from build123d import *

# Parameters (mm, degrees)
SKETCH1_W                = 20
SKETCH1_H                = 30
BOSS_EXTRUDE1_DEPTH      = 10
BOSS_EXTRUDE2_DEPTH      = 20
BOSS_EXTRUDE2_DEPTH_BACK = 20
SKETCH2_R                = 2
BOSS_EXTRUDE3_DEPTH      = 5.08
BOSS_EXTRUDE3_DEPTH_BACK = 5.08
SKETCH4_R                = 2.413
SKETCH5_W                = 5.08
SKETCH5_H                = 10
CUT_EXTRUDE1_DEPTH       = 35.777069342


with BuildPart() as part:
    # Sketch1 → Boss-Extrude1 (new body)
    with BuildSketch(Plane(origin=(0, 0, 0), x_dir=(1, 0, 0), z_dir=(0, 1, 0))):
        Rectangle(SKETCH1_W, SKETCH1_H)
    extrude(amount=BOSS_EXTRUDE1_DEPTH)

    # Sketch2 → Boss-Extrude2 (add, two sides: drawn at the far end of the back side and taken through both)
    with BuildSketch(Plane.XY.offset(-BOSS_EXTRUDE2_DEPTH_BACK)):
        with Locations((0, 5)):
            Circle(SKETCH2_R)
    extrude(amount=BOSS_EXTRUDE2_DEPTH + BOSS_EXTRUDE2_DEPTH_BACK)

    # Sketch4 → Boss-Extrude3 (add, two sides: drawn at the far end of the back side and taken through both)
    with BuildSketch(Plane(origin=(0, 0, 0), x_dir=(0, 0, -1), z_dir=(1, 0, 0)).offset(-BOSS_EXTRUDE3_DEPTH_BACK)):
        with BuildLine():
            Line((-27, 9.826), (-20, 9.826))
            Line((-20, 9.826), (-20, 0.174))
            Line((-20, 0.174), (-27, 0.174))
            ThreePointArc((-27, 0.174), (-31.826, 5), (-27, 9.826))
        make_face()
        with Locations((-27, 5)):
            Circle(SKETCH4_R, mode=Mode.SUBTRACT)
    extrude(amount=BOSS_EXTRUDE3_DEPTH + BOSS_EXTRUDE3_DEPTH_BACK)

    # Sketch5 → Cut-Extrude1 (cut, through all)
    with BuildSketch(Plane(origin=(0, 9.826, 0), x_dir=(1, 0, 0), z_dir=(0, 1, 0))):
        with Locations((0, -26.826)):
            Rectangle(SKETCH5_W, SKETCH5_H)
    extrude(amount=-CUT_EXTRUDE1_DEPTH, mode=Mode.SUBTRACT)


solid = part.part
Verification items for the finished model (mm, model axes). A direction names the side the tool comes from. Give positions to 0.01 mm unless a question says otherwise; leave off trailing zeros. Loops run counter-clockwise (first coordinate to the right, second up) from the corner with the lowest first, then second, coordinate; pieces in that order, holes last.
1) Depth check by flat-ended pin: pin 1 Ø1.5 at (x, z) = (4.5, -14.5) entering from -Y; pin 2 Ø2 at (x, z) = (-1.5, 22) entering from -Y; pin 3 Ø4 at (y, z) = (7, 19.5) entering from +X; pin 4 Ø3 at (y, z) = (3, 27) entering from -X. Enter the tip coordinate at first touch or a pass-through.
2) Thickness scan on line 1 along Z through (x, y) = (3.35, 5); line 2 along Y through (x, z) = (-4.1, 27); line 3 along X through (y, z) = (1, 22.5). Record the ranges inside material, lowest first.
3) Sectioned sample at A-A, the plane y = 3.5. Enter the section's corners in (x, z).
4) Set-up check for faces 1 (the flat face through (-5.08, 6.1, 24.5)), 2 (the flat face through (0, 0.174, 21)), 3 (the flat face through (-0.1, 7.2, 20)), 4 (the flat face through (-2.54, 6.14, 24.67)), 5 (the flat face through (0, 9.826, 21)): record each of +Z, -Z, +X, -X, +Y, -Y from which the full face is reachable in a straight line by a thin tool's end or side.
5) Sectioned sample at C-C, the plane y = 1. Enter the section's corners in (x, z).
6) Sectioned sample at B-B, the plane z = 26. Enter the section's corners in (x, y).
7) Draft check along Z on faces 6 (the cylindrical face through (0, 7, -18)), 7 (the flat face through (0, 5, 21.826)), 8 (the cylindrical face through (0, 7, 17)). Enter one of: pulls with the +Z half, pulls with the -Z half, needs draft (parallel to the pull), parting line crosses it, or undercut.
8) Sectioned sample at D-D, the plane x = 0.5. Enter the section's corners in (y, z).
Answers:
1. pin 1: stops at y = 0
1. pin 2: stops at y = 0.17
1. pin 3: stops at x = 5.08
1. pin 4: stops at x = -5.08
2. line 1: z = -15 to 15, 20 to 24.59, 29.41 to 31.83
2. line 2: y = 0.17 to 2.59, 7.41 to 9.83
2. line 3: x = -5.08 to -2.54, 2.54 to 5.08
3. outline: (-10, -15) - (-1.32, -15) - (-1.32, -20) - (1.32, -20) - (1.32, -15) - (10, -15) - (10, 15) - (1.32, 15) - (1.32, 20) - (5.08, 20) - (5.08, 25.11) - (2.54, 25.11) - (2.54, 21.83) - (-2.54, 21.83) - (-2.54, 25.11) - (-5.08, 25.11) - (-5.08, 20) - (-1.32, 20) - (-1.32, 15) - (-10, 15) - close; (-5.08, 28.89) - (-2.54, 28.89) - (-2.54, 31.59) - (-5.08, 31.59) - close; (2.54, 28.89) - (5.08, 28.89) - (5.08, 31.59) - (2.54, 31.59) - close
4. face 1: +Z, -X, +Y, -Y
4. face 2: +Z, +X, -X, -Y
4. face 3: none
4. face 4: +Z, +Y, -Y
4. face 5: +Z, +X, -X, +Y
5. outline: (-10, -15) - (10, -15) - (10, 15) - (-10, 15) - close; (-5.08, 20) - (5.08, 20) - (5.08, 29.7) - (2.54, 29.7) - (2.54, 21.83) - (-2.54, 21.83) - (-2.54, 29.7) - (-5.08, 29.7) - close
6. outline: (-5.08, 0.17) - (-2.54, 0.17) - (-2.54, 2.8) - (-5.08, 2.8) - close; (-5.08, 7.2) - (-2.54, 7.2) - (-2.54, 9.83) - (-5.08, 9.83) - close; (2.54, 0.17) - (5.08, 0.17) - (5.08, 2.8) - (2.54, 2.8) - close; (2.54, 7.2) - (5.08, 7.2) - (5.08, 9.83) - (2.54, 9.83) - close
7. face 6: needs draft
7. face 7: pulls with the +Z half
7. face 8: undercut
8. outline: (0, -15) - (3.06, -15) - (3.06, -20) - (6.94, -20) - (6.94, -15) - (10, -15) - (10, 15) - (6.94, 15) - (6.94, 20) - (9.83, 20) - (9.83, 21.83) - (0.17, 21.83) - (0.17, 20) - (3.06, 20) - (3.06, 15) - (0, 15) - close
